Part model, mm, in its own coordinate system. Face numbers are marked on the shaded views. A direction names the side the tool comes from. Give positions to 0.01 mm unless a question says otherwise; leave off trailing zeros. Order: outer loops, then holes, each group sorted by start corner. A loop starts at its lowest first (then second) coordinate and runs counter-clockwise, first axis right, second up. Notation, with made-up numbers: (23, 42) - (39, 42) arc R15 ccw to (39, 70) - close; hole circle Ø10 at (6.5, -15.75). An arc over 180 degrees is marked (long way). Use one line per item in the form item = value. Start each with the question number.
1. Band-saw the part on B-B, the plane y = 40. List the corners of the cut face in (x, z).
2. Band-saw the part on D-D, the plane x = 5.08. List the corners of the cut face in (y, z).
3. Tool access for the marked faces 4, 5 and 6: list every direction of +Z, -Z, +X, -X, +Y, -Y with a clear straight run to the whole face (end or side of a thin tool).
4. Pull direction X, two halves, no side cores. Call the marked faces 1, 2 and 3: +X half, -X half, draft (parallel to the pull), parting line (faces both ways), or undercut.
5. Drill centre lines: line 1 (Y direction, x = -5.08, z = 3.35); line 2 (Y direction, x = 3, z = 2.2); line 3 (Y direction, x = 6, z = 2.55). Where is each one in solid material? Low to high.
6. Band-saw the part on A-A, the plane x = -8.5. List the corners of the cut face in (y, z).
7. Band-saw the part on C-C, the plane y = 60.96. List the corners of the cut face in (x, z), plus the area to 3 significant figures.
8. Pin check, flat tips, straight feed: P1, Ø12, axis at x = 10.5, y = 53, coming from the -Z side; P2, Ø1.8, axis at y = -2, z = 4, coming from the -X side (3 decimals); P3, Ø1.5, axis at x = -8.5, y = 26, coming from the -Z side. Stop position of each tip, or through.
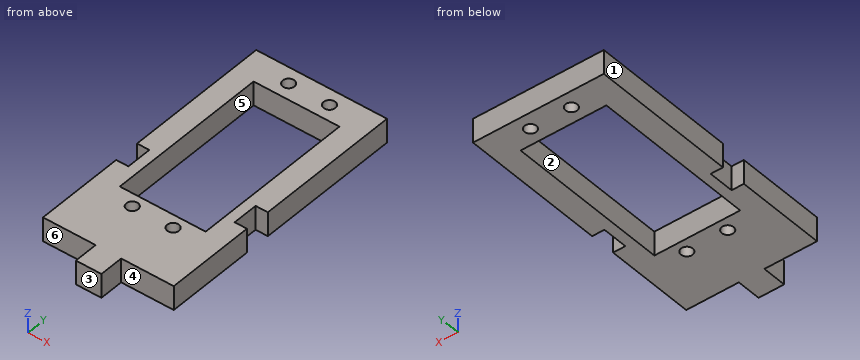
from build123d import *

# Parameters (mm, degrees)
SKETCH1_R           = 1.4605
SKETCH1_W           = 21.336
SKETCH1_H           = 40.64
BOSS_EXTRUDE1_DEPTH = 5.9944


with BuildPart() as part:
    # Sketch1 → Boss-Extrude1 (new body)
    with BuildSketch(Plane.XY):
        Polygon((-3.175, -5.9944), (3.175, -5.9944), (3.175, 0), (16.256, 0), (16.256, 22.225), (13.208, 22.225), (13.208, 28.575), (16.256, 28.575), (16.256, 64.77), (-16.256, 64.77), (-16.256, 28.575), (-13.208, 28.575), (-13.208, 22.225), (-16.256, 22.225), (-16.256, 0), (-3.175, 0), align=None)
        with Locations((5.08, 60.96)):
            Circle(SKETCH1_R, mode=Mode.SUBTRACT)
        with Locations((5.08, 13.462)):
            Circle(SKETCH1_R, mode=Mode.SUBTRACT)
        with Locations((-5.08, 13.462)):
            Circle(SKETCH1_R, mode=Mode.SUBTRACT)
        with Locations((-5.08, 60.96)):
            Circle(SKETCH1_R, mode=Mode.SUBTRACT)
        with Locations((0, 36.83)):
            Rectangle(SKETCH1_W, SKETCH1_H, mode=Mode.SUBTRACT)
    extrude(amount=BOSS_EXTRUDE1_DEPTH)


solid = part.part
From the geometry:
q1.outline = (-16.26, 0) - (-10.67, 0) - (-10.67, 5.99) - (-16.26, 5.99) - close; (10.67, 0) - (16.26, 0) - (16.26, 5.99) - (10.67, 5.99) - close
q2.outline = (0, 0) - (12, 0) - (12, 5.99) - (0, 5.99) - close; (14.92, 0) - (16.51, 0) - (16.51, 5.99) - (14.92, 5.99) - close; (57.15, 0) - (59.5, 0) - (59.5, 5.99) - (57.15, 5.99) - close; (62.42, 0) - (64.77, 0) - (64.77, 5.99) - (62.42, 5.99) - close
q3.face_4 = +Z, -Z, +X, -Y
q3.face_5 = +Z, -Z
q3.face_6 = +Z, -Z, -X, -Y
q4.face_1 = -X half
q4.face_2 = undercut
q4.face_3 = draft
q5.line_1 = 0 to 12, 14.92 to 16.51, 57.15 to 59.5, 62.42 to 64.77
q5.line_2 = -5.99 to 16.51, 57.15 to 64.77
q5.line_3 = 0 to 12.33, 14.6 to 16.51, 57.15 to 59.83, 62.09 to 64.77
q6.outline = (0, 0) - (16.51, 0) - (16.51, 5.99) - (0, 5.99) - close; (57.15, 0) - (64.77, 0) - (64.77, 5.99) - (57.15, 5.99) - close
q7.outline = (-16.26, 0) - (-6.54, 0) - (-6.54, 5.99) - (-16.26, 5.99) - close; (-3.62, 0) - (3.62, 0) - (3.62, 5.99) - (-3.62, 5.99) - close; (6.54, 0) - (16.26, 0) - (16.26, 5.99) - (6.54, 5.99) - close
q7.area = 160 mm²
q8.P1 = 0
q8.P2 = -3.175
q8.P3 = through
